```python
from build123d import *

# Parameters (mm, degrees)
SKETCH1_R           = 1.55
BOSS_EXTRUDE1_DEPTH = 1
CHAMFER1_SIZE       = 1.5
SKETCH5_W           = 9.75
SKETCH5_H           = 17.3
SKETCH5_H_2         = 5
BOSS_EXTRUDE2_DEPTH = 2.2
FILLET2_R           = 5


with BuildPart() as part:
    # Sketch1 → Boss-Extrude1 (new body)
    with BuildSketch(Plane(origin=(0, 0, 0), x_dir=(1, 0, 0), z_dir=(0, 1, 0))):
        with BuildLine():
            Line((-11.55, 10), (-16.5, 10))
            Line((-16.5, 10), (-16.5, 12))
            Line((-16.5, 12), (-26.25, 12))
            Line((-26.25, 12), (-26.25, -14))
            ThreePointArc((-26.25, -14), (-25.957106781, -14.707106781), (-25.25, -15))
            Line((-25.25, -15), (-22.25, -15))
            ThreePointArc((-22.25, -15), (-21.542893219, -14.707106781), (-21.25, -14))
            Line((-21.25, -14), (-21.25, -10))
            Line((-21.25, -10), (21.25, -10))
            Line((21.25, -10), (21.25, -14))
            ThreePointArc((21.25, -14), (21.542893219, -14.707106781), (22.25, -15))
            Line((22.25, -15), (25.25, -15))
            ThreePointArc((25.25, -15), (25.957106781, -14.707106781), (26.25, -14))
            Line((26.25, -14), (26.25, 12))
            Line((26.25, 12), (16.5, 12))
            Line((16.5, 12), (16.5, 10))
            Line((16.5, 10), (9.05, 10))
            ThreePointArc((9.05, 10), (8.484314575, 9.765685425), (8.25, 9.2))
            Line((8.25, 9.2), (8.25, 9))
            ThreePointArc((8.25, 9), (7.957106781, 8.292893219), (7.25, 8))
            Line((7.25, 8), (-9.75, 8))
            ThreePointArc((-9.75, 8), (-10.457106781, 8.292893219), (-10.75, 9))
            Line((-10.75, 9), (-10.75, 9.2))
            ThreePointArc((-10.75, 9.2), (-10.984314575, 9.765685425), (-11.55, 10))
        make_face()
        with BuildLine():
            Line((6.25, -5), (-8.75, -5))
            ThreePointArc((-8.75, -5), (-10.164213562, -4.414213562), (-10.75, -3))
            Line((-10.75, -3), (-10.75, 3))
            ThreePointArc((-10.75, 3), (-10.164213562, 4.414213562), (-8.75, 5))
            Line((-8.75, 5), (6.25, 5))
            ThreePointArc((6.25, 5), (7.664213562, 4.414213562), (8.25, 3))
            Line((8.25, 3), (8.25, -3))
            ThreePointArc((8.25, -3), (7.664213562, -4.414213562), (6.25, -5))
        make_face(mode=Mode.SUBTRACT)
        with Locations(Location((-23.75, -12.5, 0), (0, 0, 270))):
            Circle(SKETCH1_R, mode=Mode.SUBTRACT)
        with Locations(Location((23.75, -12.5, 0), (0, 0, 270))):
            Circle(SKETCH1_R, mode=Mode.SUBTRACT)
    extrude(amount=BOSS_EXTRUDE1_DEPTH)

    # Chamfer1
    # the kernel refuses this chamfer: 1.5 mm, written as the material it takes off along each edge
    with BuildSketch(Plane(origin=(-12.642475518, 1, -12), x_dir=(0, -0.9996219169112968, -0.027495876610586778), z_dir=(-1, 0, 0)), Plane(origin=(30.107524482, 1, -12), x_dir=(0, -0.9996219169112968, -0.027495876610586778), z_dir=(-1, 0, 0))) as chamfer1_piece_1:
        Polygon((CHAMFER1_SIZE * 0.999621916911, CHAMFER1_SIZE * 0.0274958766106), (-CHAMFER1_SIZE * 0.0274958766106, CHAMFER1_SIZE * 0.999621916911), (0, 0), align=None)
    extrude(amount=17.465048964, mode=Mode.SUBTRACT)

    # Sketch5 → Boss-Extrude2 (add)
    with BuildSketch(Plane.XZ):
        with Locations((-21.375, -0.25)):
            Rectangle(SKETCH5_W, SKETCH5_H)
        with Locations((21.375, 2.8)):
            Rectangle(SKETCH5_W, SKETCH5_H_2)
    extrude(amount=BOSS_EXTRUDE2_DEPTH)

    # Fillet2
    fillet2_edges = [part.edges().sort_by_distance(p)[0] for p in [
        (21.25, 0.5, 10),
        (-21.25, 0.5, 10),
    ]]
    fillet(fillet2_edges, radius=FILLET2_R)


solid = part.part
```
For this review, take the finished solid that the model builds, in its own axes (mm). A direction names the side the tool comes from. Coordinates: 2 decimals unless noted, no trailing zeros. Loops run counter-clockwise (first coordinate to the right, second up) from the corner with the lowest first, then second, coordinate; pieces in that order, holes last. Notation, with made-up numbers: (34.25, 31.25) -> (79.25, 31.25) arc R13 ccw to (79.25, 46.25) -> close; hole circle Ø9 at (61.5, -32.75). An arc over 180 degrees is marked (long way). Return JSON: item names as keys, results as strings. Group by question number.
(1) For pin 1 Ø1.1 at (x, y) = (20, -1.5) entering from -Z; pin 2 Ø1.8 at (x, y) = (-22, -1) entering from +Z; pin 3 Ø1.1 at (x, y) = (22.5, -1.5) entering from +Z, all flat-tipped, find the tip position at first contact; note any pin that passes through.
(2) Consider section B-B, the plane x = 23.75. Give the boundary of the cut face in (y, z).
(3) Consider section A-A, the plane z = 2.5. Give the boundary of the cut face in (x, y), plus the area to 3 significant figures.
(4) To check wall thickness, follow L1, parallel to X at y = 0.7, z = 12.5; L2, parallel to X at y = -1.6, z = 4.75; L3, parallel to Z at x = 0, y = 0.3. State the ranges of each line that lie inside material, in increasing order.
(5) Consider section C-C, the plane x = -6. Give the boundary of the cut face in (y, z), plus the area to 3 significant figures.
(6) Mouldability with a two-part tool opening along Z and no side actions: class faces 1 (the flat face through (-23.8, 0.5, 15)), 2 (the cylindrical face through (-10.15, 0.49, 4.43)), 3 (the flat face through (21.4, 0.5, -11)), 4 (the flat face through (5, 0, -7)) as pulls with the +Z half, pulls with the -Z half, needs draft (parallel to the pull), parting line crosses it, or undercut.
(7) Consider section D-D, the plane z = 7.75. Give the boundary of the cut face in (x, y).
(8) Tool access review of faces 5 (the flat face through (-1.4, 0.5, -5)), 6 (the cylindrical face through (-21.61, 0.49, 14.77)), 7 (the flat face through (-16.5, -1, 0)), 8 (the cylindrical face through (-10.449, 0.493, -8.285)): name each direction out of +Z, -Z, +X, -X, +Y, -Y from which nothing blocks a thin tool from reaching the whole face with its end or side.
Results below:
{
 "1": {"pin 1": "stops at z = 0.3", "pin 2": "stops at z = 8.4", "pin 3": "stops at z = 5.3"},
 "2": {"outline": "(-2.2, 0.3) -> (0, 0.3) -> (0, -11.5) -> (1, -10.5) -> (1, 10.95) -> (0, 10.95) -> (0, 5.3) -> (-2.2, 5.3) -> close; (0, 14.05) -> (1, 14.05) -> (1, 15) -> (0, 15) -> close"},
 "3": {"outline": "(-26.25, -2.2) -> (-16.5, -2.2) -> (-16.5, 0) -> (-10.75, 0) -> (-10.75, 1) -> (-26.25, 1) -> close; (8.25, 0) -> (16.5, 0) -> (16.5, -2.2) -> (26.25, -2.2) -> (26.25, 1) -> (8.25, 1) -> close", "area": "76.4 mm2"},
 "4": {"L1": "x = -26.25 to -25.3, -22.2 to -20.66, 20.66 to 22.2, 25.3 to 26.25", "L2": "x = -26.25 to -16.5, 16.5 to 26.25", "L3": "z = -8 to -5, 5 to 10"},
 "5": {"outline": "(0, -8) -> (1, -8) -> (1, -5) -> (0, -5) -> close; (0, 5) -> (1, 5) -> (1, 10) -> (0, 10) -> close", "area": "8.00 mm2"},
 "6": {"face 1": "pulls with the +Z half", "face 2": "undercut", "face 3": "pulls with the -Z half", "face 4": "needs draft"},
 "7": {"outline": "(-26.25, -2.2) -> (-16.5, -2.2) -> (-16.5, 0) -> (26.25, 0) -> (26.25, 1) -> (-26.25, 1) -> close"},
 "8": {"face 5": "+Y, -Y", "face 6": "+Z, +Y, -Y", "face 7": "+Z, -Z, -Y", "face 8": "-Z, +Y, -Y"}
}
